Autodesk Inventor part; units mm, degrees
ref_plane "YZ Plane" through (0, 0, 0) normal (1, 0, 0) x (0, 1, 0)
ref_plane "XZ Plane" through (0, 0, 0) normal (0, 1, 0) x (-1, 0, 0)
ref_plane "XY Plane" through (0, 0, 0) normal (0, 0, 1) x (1, 0, 0)
sketch "Sketch1" plane through (0, 0, 0) normal (0, 1, 0) x (-1, 0, 0)
  line L0 (0, 0) -> (42.3, 0)
  line L1 (42.3, 0) -> (42.3, 42.3)
  line L2 (42.3, 42.3) -> (0, 42.3)
  line L3 (0, 42.3) -> (0, 0)
  dimension "d0" = 42.3
  dimension "d1" = 42.3
extrude "Extrusion1" add sketch "Sketch1" along normal blind 40
sketch "Sketch2" plane through (0, 40, 0) normal (0, 1, 0) x (1, 0, 0)
  line L0 (0, 0) -> (-42.3, 0)
  line L1 (0, -42.3) -> (0, 0)
  circle A0 centre (-21.15, -21.15) radius 11
  point P0 (0, -2)
  point P1 (-2, 0)
  point P2 (-40.3, 0)
  point P3 (0, -40.3)
  dimension "d6" = 22
  dimension "d7" = 21.15
  dimension "d8" = 21.15
extrude "Extrusion2" add sketch "Sketch2" along normal blind 2
sketch "Sketch3" plane through (-21.15, 42, 21.15) normal (0, 1, 0) x (1, 0, 0)
  circle A0 centre (0, 0) radius 11
  circle A1 centre (0, 0) radius 2.5
  point P0 (21.15, 21.15)
  dimension "d11" = 5
extrude "Extrusion3" add sketch "Sketch3" along normal blind 22 contours A1
sketch "Sketch4" plane through (-21.15, 64, 21.15) normal (0, 1, 0) x (1, 0, 0)
  circle A0 centre (0, 0) radius 2.5
  line L0 (-1.5, 2) -> (1.5, 2)
  point P0 (21.15, 21.15)
  dimension "d14" = 2
extrude "Extrusion4" cut sketch "Sketch4" against normal blind 21 contours L0 A0 picked at (-0.3466, 2.0912)
sketch "Sketch5" plane through (0, 40, 0) normal (0, 1, 0) x (1, 0, 0)
  line L0 (-42.3, 0) -> (-42.3, -42.3)
  line L1 (-42.3, -42.3) -> (0, -42.3)
  circle A0 centre (-36.65, -5.65) radius 1.5
  circle A1 centre (-5.65, -5.65) radius 1.5
  circle A2 centre (-5.65, -36.65) radius 1.5
  circle A3 centre (-36.65, -36.65) radius 1.5
  point P0 (-42.3, -2)
  point P1 (-42.3, -40.3)
  point P2 (-40.3, -42.3)
  point P3 (-2, -42.3)
  point P4 (0, 0)
  dimension "d17" = 3
  dimension "d18" = 3
  dimension "d19" = 3
  dimension "d20" = 3
  dimension "d21" = 31
  dimension "d22" = 5.65
  dimension "d23" = 31
  dimension "d24" = 5.65
extrude "Extrusion5" cut sketch "Sketch5" against normal blind 4.5
chamfer "Chamfer1" distance 4 angle 45 4 edges at (-42.3, 20, 0) (-42.3, 20, 42.3) (0, 20, 0) (0, 20, 42.3)
properties part number "StepperMotorNema17x40mm"
The model under review builds one solid part; all positions refer to its coordinate system, in mm. A direction names the side the tool comes from. Round coordinates to 2 decimals unless told otherwise and drop trailing zeros. Order: outer loops, then holes, each group sorted by start corner. A loop starts at its lowest first (then second) coordinate and runs counter-clockwise, first axis right, second up. Notation, with made-up numbers: M 25,6 L 79,6 A12 cw 79,19 Z; hole C 35,-19 d4. An arc over 180 degrees is marked long. Use a Markdown table: item, result.
1) Consider section B-B (z = 5.65). Write out the cut boundary in (x, y).
Report:
| item | result |
|---|---|
| outline | M -42.3,0 L 0,0 L 0,40 L -4.15,40 L -4.15,35.5 L -7.15,35.5 L -7.15,40 L -35.15,40 L -35.15,35.5 L -38.15,35.5 L -38.15,40 L -42.3,40 Z |
2) Wall thickness on line 1 along Z through (x, y) = (-36.65, 39.15); line 2 along X through (y, z) = (37.1, 5.65); line 3 along Z through (x, y) = (-5, 37): over which ranges is each line inside the solid? List them lowest first. Write a range as [from, to].
Report:
| item | result |
|---|---|
| line 1 | [0, 4.15], [7.15, 35.15], [38.15, 42.3] |
| line 2 | [-42.3, -38.15], [-35.15, -7.15], [-4.15, 0] |
| line 3 | [0, 4.3], [7, 35.3], [38, 42.3] |
3) Consider section D-D (x = -36.65). Write out the cut boundary in (y, z), then the cut area to 4 significant figures.
Report:
| item | result |
|---|---|
| outline | M 0,0 L 40,0 L 40,4.15 L 35.5,4.15 L 35.5,7.15 L 40,7.15 L 40,35.15 L 35.5,35.15 L 35.5,38.15 L 40,38.15 L 40,42.3 L 0,42.3 Z |
| area | 1,665 mm^2 |
4) Insertion check: pin 1 (2.5 mm diameter, centred on x = -36.5, z = 6, fed in from +Y); pin 2 (0.9 mm diameter, centred on x = -37, z = 36, fed in from +Y); pin 3 (8 mm diameter, centred on x = -22.5, y = 46.5, fed in from +Z). Each pin has a flat end and moves straight along its axis. Give the tip position at first contact, or say it passes through.
Report:
| item | result |
|---|---|
| pin 1 | y = 40 |
| pin 2 | y = 35.5 |
| pin 3 | z = 23.65 |
5) Draft analysis for pull direction X (two halves, no side actions). For faces 4 (the face through (-42.3, 20, 21)), 5 (the face through (-38.15, 37.78, 5.58)), 6 (the face through (-21, 0, 21)), state which applies: released by +X, released by -X, zero draft, split by the parting line, or undercut.
Report:
| item | result |
|---|---|
| face 4 | released by -X |
| face 5 | undercut |
| face 6 | zero draft |
6) Tool access review of faces 1 (the face through (-21, 54, 19.15)), 2 (the face through (-37.84, 37.78, 37.56)), 3 (the face through (0, 20, 21)): name each direction out of +Z, -Z, +X, -X, +Y, -Y from which nothing blocks a thin tool from reaching the whole face with its end or side.
Report:
| item | result |
|---|---|
| face 1 | -Z, +X, -X, +Y |
| face 2 | +Y |
| face 3 | +Z, -Z, +X, +Y, -Y |
7) Consider section C-C (y = 8). Write out the cut boundary in (x, z).
Report:
| item | result |
|---|---|
| outline | M -42.3,4 L -38.3,0 L -4,0 L 0,4 L 0,38.3 L -4,42.3 L -38.3,42.3 L -42.3,38.3 Z |
8) Consider section A-A (x = -21.15). Write out the cut boundary in (y, z).
Report:
| item | result |
|---|---|
| outline | M 0,0 L 40,0 L 40,10.15 L 42,10.15 L 42,18.65 L 43,18.65 L 43,19.15 L 64,19.15 L 64,23.65 L 42,23.65 L 42,32.15 L 40,32.15 L 40,42.3 L 0,42.3 Z |
